Design review of the part built by this model. Coordinates are the model's own, in mm. Coordinates: 2 decimals unless noted, no trailing zeros. Use CSV: the item, a comma, the result in double quotes.
```python
from build123d import *

# Parameters (mm, degrees)
SKETCH_1_W          = 180
SKETCH_1_H          = 130
EXTRUDE_1_DEPTH     = 3
FILLET_1_R          = 10
SKETCH_2_R          = 3.5
CUT_EXTRUDE_1_DEPTH = 112.05854312


with BuildPart() as part:
    # 草图1 → 凸台-拉伸1 (new body)
    with BuildSketch(Plane.XY):
        Rectangle(SKETCH_1_W, SKETCH_1_H)
    extrude(amount=EXTRUDE_1_DEPTH)

    # 圆角1
    fillet_1_edges = [part.edges().sort_by_distance(p)[0] for p in [
        (90, -65, 1.5),
        (-90, -65, 1.5),
        (-90, 65, 1.5),
        (90, 65, 1.5),
    ]]
    fillet(fillet_1_edges, radius=FILLET_1_R)

    # 草图2 → 切除-拉伸1 (cut, through all)
    with BuildSketch(Plane.XY.offset(3)):
        with Locations((-80, 55)):
            Circle(SKETCH_2_R)
        with Locations((-80, -55)):
            Circle(SKETCH_2_R)
        with Locations((80, 55)):
            Circle(SKETCH_2_R)
        with Locations((80, -55)):
            Circle(SKETCH_2_R)
    extrude(amount=-CUT_EXTRUDE_1_DEPTH, mode=Mode.SUBTRACT)


solid = part.part
```
Item 1: To check wall thickness, follow line 1 along Y through (x, z) = (-80, 1.7); line 2 along X through (y, z) = (-52.5, 0.55). State the ranges of each line that lie inside material, in increasing order.
Checked values:
line 1,"-65 to -58.5, -51.5 to 51.5, 58.5 to 65"
line 2,"-90 to -82.45, -77.55 to 77.55, 82.45 to 90"
Item 2: Draft analysis for pull direction X (two halves, no side actions). For faces 1 (the face through (87.15, 61.99, 1.52)), 2 (the face through (-1, 1, 3)), 3 (the face through (-87.15, 61.99, 1.52)), 4 (the face through (83.34, 56.05, 1.52)), state which applies: pulls with the +X half, pulls with the -X half, needs draft (parallel to the pull), parting line crosses it, or undercut.
Checked values:
face 1,"pulls with the +X half"
face 2,"needs draft"
face 3,"pulls with the -X half"
face 4,"undercut"
Item 3: Clearance check with a flat-ended pin moving along its axis: pin 1 (5.5 mm diameter, centred on x = 80, y = 55, fed in from -Z). State where the tip first meets the part, or that it passes through.
Checked values:
pin 1,"through"
